Can you work these out from the model? Positions are in its coordinate system, mm. A direction names the side the tool comes from. Give positions to 0.01 mm unless a question says otherwise; leave off trailing zeros. Loops run counter-clockwise (first coordinate to the right, second up) from the corner with the lowest first, then second, coordinate; pieces in that order, holes last.
Autodesk Inventor part; units mm, degrees
ref_plane "YZ Plane" through (0, 0, 0) normal (1, 0, 0) x (0, 1, 0)
ref_plane "XZ Plane" through (0, 0, 0) normal (0, 1, 0) x (-1, 0, 0)
ref_plane "XY Plane" through (0, 0, 0) normal (0, 0, 1) x (1, 0, 0)
sketch "Sketch1" plane through (0, 0, 0) normal (0, 1, 0) x (-1, 0, 0)
  line L0 (0, 0) -> (12.3, 0)
  circle A0 centre (12.3, 0) radius 9.65
  circle A1 centre (12.3, 0) radius 6
  arc A2 (12.3, -14) -> (12.3, 14) centre (12.3, 0) ccw
  line L1 (12.3, 14) -> (0, 14)
  line L2 (0, 14) -> (0, 24)
  line L3 (0, 24) -> (6, 24)
  line L4 (6, 24) -> (6, 14)
  line L5 (12.3, -14) -> (0, -14)
  line L6 (0, -14) -> (0, -24)
  line L7 (0, -24) -> (6, -24)
  line L8 (6, -24) -> (6, -14)
  line L9 (0, 14) -> (0, -14)
  dimension "d0" = 12.3
  dimension "d1" = 19.3
  dimension "d2" = 12
  dimension "d3" = 28
  dimension "d4" = 10
  dimension "d5" = 6
  dimension "d6" = 10
extrude "Extrusion1" add sketch "Sketch1" along normal blind 3 contours A0
extrude "Extrusion2" add sketch "Sketch1" along normal blind 9 contours L9 L1 A2 L5 | L2 L3 L4 L1 | L5 L8 L7 L6
sketch "Sketch2" plane through (0, 0, 24) normal (1, 0, 0) x (0, 0, -1)
  line L0 (0, 0) -> (0, 9)
  line L1 (0, 4.5) -> (5, 4.5)
  line L2 (48, 0) -> (48, 9)
  line L3 (48, 4.5) -> (43, 4.5)
  circle A0 centre (5, 4.5) radius 2.6
  circle A1 centre (43, 4.5) radius 2.6
  point P0 (24, 0)
  dimension "d11" = 5
  dimension "d12" = 5
  dimension "d13" = 5.2
  dimension "d14" = 5.2
extrude "Extrusion3" cut sketch "Sketch2" against normal blind 9
properties part number "bearing_holder_plate_tb"
(1) Suppose I cut it at C-C on x = -5. List the corners of the cut face in (y, z) for me, plus the area to 3 significant figures.
Returned:
outline: (0, -24) - (9, -24) - (9, -6.31) - (3, -6.31) - (3, 6.31) - (9, 6.31) - (9, 24) - (0, 24) - close; hole circle Ø5.2 at (4.5, -19); hole circle Ø5.2 at (4.5, 19)
area: 314 mm2
(2) Please list where these lines run through material, in increasing order: probe 1 along Y at (x, z) = (-5.75, 19); probe 2 along Z at (x, y) = (-12.3, 7); probe 3 along Z at (x, y) = (-12.3, 1.1).
Returned:
probe 1: y = 0 to 1.9, 7.1 to 9
probe 2: z = -14 to -9.65, 9.65 to 14
probe 3: z = -14 to -6, 6 to 14
(3) Suppose I cut it at D-D on z = -8.5. List the corners of the cut face in (x, y) for me.
Returned:
outline: (-23.42, 0) - (0, 0) - (0, 9) - (-7.73, 9) - (-7.73, 3) - (-16.87, 3) - (-16.87, 9) - (-23.42, 9) - close
(4) Which directions (+Z, -Z, +X, -X, +Y, -Y) give clear straight access to the entire face, cutting with the end or side of a thin tool? Please do faces 4 (the cylindrical face through (-2.96, 5.28, -21.48)), 5 (the flat face through (-9, 4, -14)), 6 (the flat face through (-6, 6.4, 21.3)).
Returned:
face 4: +X, -X
face 5: -Z, -X, +Y, -Y
face 6: +Z, -X, +Y, -Y
(5) Suppose I cut it at B-B on z = -19. List the corners of the cut face in (x, y) for me.
Returned:
outline: (-6, 0) - (0, 0) - (0, 1.9) - (-6, 1.9) - close; (-6, 7.1) - (0, 7.1) - (0, 9) - (-6, 9) - close
(6) Will these pins go through, and if not, where does the flat tip stop? P1, Ø3, axis at x = -16, y = 4.5, coming from the +Z side; P2, Ø6, axis at x = -21, z = 11, coming from the -Y side; P3, Ø15.5, axis at x = -13, z = 1, coming from the +Y side; P4, Ø3, axis at x = -8, y = 6.5, coming from the +Z side.
Returned:
P1: stops at z = 13.83
P2: stops at y = 0
P3: stops at y = 3
P4: stops at z = 14
(7) Thinking about a two-plate mould opening in Y: for faces 1 (the flat face through (-12.2, 3, -6.3)), 2 (the cylindrical face through (-2.66, 5.96, -0.42)), 3 (the cylindrical face through (-2.96, 5.28, 16.52)), which applies, pulls with the +Y half, pulls with the -Y half, needs draft (parallel to the pull), parting line crosses it, or undercut?
Returned:
face 1: pulls with the +Y half
face 2: needs draft
face 3: undercut
(8) Suppose I cut it at A-A on y = 5.5. List the corners of the cut face in (x, z) for me.
Returned:
outline: (-12.3, -14) - (-6, -14) - (-6, -16.6) - (0, -16.6) - (0, 16.6) - (-6, 16.6) - (-6, 14) - (-12.3, 14) arc R14 ccw to start; (-6, -24) - (0, -24) - (0, -21.4) - (-6, -21.4) - close; (-6, 21.4) - (0, 21.4) - (0, 24) - (-6, 24) - close; hole circle Ø19.3 at (-12.3, 0)
